Could you check a few things on this model? Use its own coordinates, in mm. Round coordinates to 2 decimals unless told otherwise and drop trailing zeros. Loops run counter-clockwise (first coordinate to the right, second up) from the corner with the lowest first, then second, coordinate; pieces in that order, holes last. Notation, with made-up numbers: M -20.5,0.5 L 13.5,0.5 A9 cw 13.5,8.5 Z; hole C 49,67.25 d5. An arc over 180 degrees is marked long. One line per item, written item: value. Start each with the question number.
Q1. I'm going to push flat-ended pins straight in: pin 1 Ø2 at (x, y) = (29.5, -3) entering from -Z; pin 2 Ø7 at (x, y) = (29, 7) entering from +Z; pin 3 Ø2 at (x, y) = (15.5, -6.5) entering from -Z. Where does each tip first touch, or does it pass through?
Q2. Please list where these lines run through material, in increasing order: line 1 along Y through (x, z) = (32.5, 65); line 2 along Y through (x, z) = (26, 16.5); line 3 along X through (y, z) = (6.5, 12).
Q3. Imagine slicing it at A-A (z = 8.5). Please give me the cut outline in (x, y).
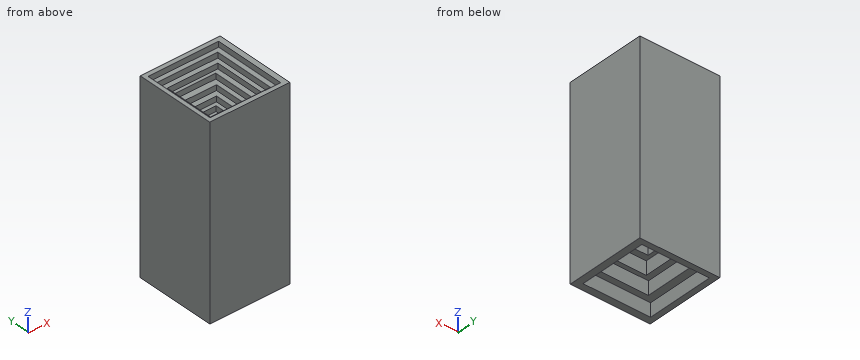
from build123d import *

# Parameters (mm, degrees)
F0_W      = 29.753645
F0_H      = 29.910467
F1_DEPTH  = 69.4
F2_W      = 26.227938
F2_H      = 26.650196
F3_DEPTH  = 2
F4_W      = 22.616781
F4_H      = 22.63493
F5_DEPTH  = 2
F6_W      = 18.798804
F6_H      = 18.714747
F7_DEPTH  = 2
F8_W      = 15.419276
F8_H      = 15.666918
F9_DEPTH  = 2
F10_W     = 12.241865
F10_H     = 11.595491
F11_DEPTH = 2
F12_W     = 8.867356
F12_H     = 8.313611
F13_DEPTH = 2
F14_W     = 5.944216
F14_H     = 5.405146
F15_DEPTH = 2
F16_W     = 3.43767
F16_H     = 2.966377
F17_DEPTH = 55.401
F18_W     = 25.107885
F18_H     = 25.31029
F19_DEPTH = 5
F20_W     = 19.709587
F20_H     = 20.623714
F21_DEPTH = 5
F22_W     = 15.688963
F22_H     = 16.865403
F23_DEPTH = 5
F24_W     = 12.248309
F24_H     = 12.584658
F25_DEPTH = 5
F26_W     = 8.523883
F26_H     = 8.044946
F27_DEPTH = 5
F28_W     = 6.262533
F28_H     = 5.897496
F29_DEPTH = 5


with BuildPart() as f1:
    # F0 (on Top) → F1 (new body)
    with BuildSketch(Plane.XY):
        with Locations((26.444191, 1.299118)):
            Rectangle(F0_W, F0_H)
    extrude(amount=F1_DEPTH)

    # F2 (on face) → F3 (cut)
    with BuildSketch(Plane.XY.offset(69.4)):
        with Locations((26.172734, 1.267092)):
            Rectangle(F2_W, F2_H)
    extrude(amount=-F3_DEPTH, mode=Mode.SUBTRACT)

    # F4 (on face) → F5 (cut)
    with BuildSketch(Plane.XY.offset(67.4)):
        with Locations((26.183258, 1.558795)):
            Rectangle(F4_W, F4_H)
    extrude(amount=-F5_DEPTH, mode=Mode.SUBTRACT)

    # F6 (on face) → F7 (cut)
    with BuildSketch(Plane.XY.offset(65.4)):
        with Locations((26.503739, 1.66645)):
            Rectangle(F6_W, F6_H)
    extrude(amount=-F7_DEPTH, mode=Mode.SUBTRACT)

    # F8 (on face) → F9 (cut)
    with BuildSketch(Plane.XY.offset(63.4)):
        with Locations((26.353671, 1.952434)):
            Rectangle(F8_W, F8_H)
    extrude(amount=-F9_DEPTH, mode=Mode.SUBTRACT)

    # F10 (on face) → F11 (cut)
    with BuildSketch(Plane.XY.offset(61.4)):
        with Locations((26.306717, 1.756216)):
            Rectangle(F10_W, F10_H)
    extrude(amount=-F11_DEPTH, mode=Mode.SUBTRACT)

    # F12 (on face) → F13 (cut)
    with BuildSketch(Plane.XY.offset(59.4)):
        with Locations((26.212682, 1.37607)):
            Rectangle(F12_W, F12_H)
    extrude(amount=-F13_DEPTH, mode=Mode.SUBTRACT)

    # F14 (on face) → F15 (cut)
    with BuildSketch(Plane.XY.offset(57.4)):
        with Locations((26.353785, 1.47873)):
            Rectangle(F14_W, F14_H)
    extrude(amount=-F15_DEPTH, mode=Mode.SUBTRACT)

    # F16 (on face) → F17 (cut, through all)
    with BuildSketch(Plane.XY.offset(55.4)):
        with Locations((26.232888, 1.483189)):
            Rectangle(F16_W, F16_H)
    extrude(amount=-F17_DEPTH, mode=Mode.SUBTRACT)

    # F18 (on face) → F19 (cut)
    with BuildSketch(Plane(origin=(0, 0, 0), x_dir=(1, 0, 0), z_dir=(0, 0, -1))):
        with Locations((26.205565, -1.541603)):
            Rectangle(F18_W, F18_H)
    extrude(amount=-F19_DEPTH, mode=Mode.SUBTRACT)

    # F20 (on face) → F21 (cut)
    with BuildSketch(Plane(origin=(0, 0, 5), x_dir=(1, 0, 0), z_dir=(0, 0, -1))):
        with Locations((26.284554, -1.530935)):
            Rectangle(F20_W, F20_H)
    extrude(amount=-F21_DEPTH, mode=Mode.SUBTRACT)

    # F22 (on face) → F23 (cut)
    with BuildSketch(Plane(origin=(0, 0, 10), x_dir=(1, 0, 0), z_dir=(0, 0, -1))):
        with Locations((26.510216, -1.292301)):
            Rectangle(F22_W, F22_H)
    extrude(amount=-F23_DEPTH, mode=Mode.SUBTRACT)

    # F24 (on face) → F25 (cut)
    with BuildSketch(Plane(origin=(0, 0, 15), x_dir=(1, 0, 0), z_dir=(0, 0, -1))):
        with Locations((26.16421, -1.464862)):
            Rectangle(F24_W, F24_H)
    extrude(amount=-F25_DEPTH, mode=Mode.SUBTRACT)

    # F26 (on face) → F27 (cut)
    with BuildSketch(Plane(origin=(0, 0, 20), x_dir=(1, 0, 0), z_dir=(0, 0, -1))):
        with Locations((26.223567, -1.529857)):
            Rectangle(F26_W, F26_H)
    extrude(amount=-F27_DEPTH, mode=Mode.SUBTRACT)

    # F28 (on face) → F29 (cut)
    with BuildSketch(Plane(origin=(0, 0, 25), x_dir=(1, 0, 0), z_dir=(0, 0, -1))):
        with Locations((26.28174, -1.536325)):
            Rectangle(F28_W, F28_H)
    extrude(amount=-F29_DEPTH, mode=Mode.SUBTRACT)


solid = f1.part
Report:
1. pin 1: stops at z = 20
1. pin 2: stops at z = 63.4
1. pin 3: stops at z = 5
2. line 1: y = -13.66 to -7.69, 11.02 to 16.25
2. line 2: y = -13.66 to -4.83, 7.76 to 16.25
2. line 3: x = 11.57 to 18.67, 34.35 to 41.32
3. outline: M 11.57,-13.66 L 41.32,-13.66 L 41.32,16.25 L 11.57,16.25 Z; hole M 16.43,-8.78 L 36.14,-8.78 L 36.14,11.84 L 16.43,11.84 Z
